```python
from build123d import *

# Parameters (mm, degrees)
F0_R     = 34.798
F1_DEPTH = 6.35
F2_DEPTH = 25.4
F3_DEPTH = 101.6
F4_DEPTH = 101.6


with BuildPart() as f1:
    # F0 (on Front) → F1 (new body)
    with BuildSketch(Plane.XZ):
        Circle(F0_R)
    extrude(amount=F1_DEPTH)

    # F2 (add): a face of the model
    f2_faces = [f1.faces().sort_by_distance(p)[0] for p in [
        (0, -6.35, 0),
    ]]
    extrude(f2_faces, amount=F2_DEPTH)

    # F3 (add): a face of the model
    f3_faces = [f1.faces().sort_by_distance(p)[0] for p in [
        (0, -31.75, 0),
    ]]
    extrude(f3_faces, amount=F3_DEPTH)

    # F4 (add): a face of the model
    f4_faces = [f1.faces().sort_by_distance(p)[0] for p in [
        (0, 0, 0),
    ]]
    extrude(f4_faces, amount=F4_DEPTH)


solid = f1.part
```
Source: CAD feature listing. Evaluate the final solid. Frame: model axes, mm. Round coordinates to 2 decimals unless told otherwise and drop trailing zeros. Loops run counter-clockwise (first coordinate to the right, second up) from the corner with the lowest first, then second, coordinate; pieces in that order, holes last. Notation, with made-up numbers: M 6.5,14.25 L 17.5,14.25 A20 cw 17.5,48.25 Z; hole C 2,87 d9. An arc over 180 degrees is marked long. Use a Markdown table: item, result. Add a question column.
1. Ray query, line 1 along X through (y, z) = (75, 1); line 2 along Z through (x, y) = (-0.5, -121); line 3 along X through (y, z) = (-113, 12). Return the intervals inside material, ascending. Write a range as [from, to].
2. Cut plane C-C, the plane x = 27. Output: boundary loops of the cut face in (y, z), and give its area (3 significant figures).
3. Cut plane B-B, the plane z = 14. Output: boundary loops of the cut face in (x, y), and give its area (3 significant figures).
4. Cut plane A-A, the plane y = -66.5. Output: boundary loops of the cut face in (x, z), and give its area (3 significant figures).
5. Contact query for flat-ended pins moving along their axis: pin 1 (1.5 mm diameter, centred on x = 25, y = -107, fed in from -Z); pin 2 (8 mm diameter, centred on x = -27, y = -25.5, fed in from -Z); pin 3 (5 mm diameter, centred on y = 74, z = -10, fed in from -X). Output: stop coordinate, or through.
Solution:
| question | item | result |
|---|---|---|
| 1 | line 1 | x = [-34.78, 34.78] |
| 1 | line 2 | z = [-34.79, 34.79] |
| 1 | line 3 | x = [-32.66, 32.66] |
| 2 | outline | M -133.35,-21.95 L 101.6,-21.95 L 101.6,21.95 L -133.35,21.95 Z |
| 2 | area | 10,300 mm2 |
| 3 | outline | M -31.86,-133.35 L 31.86,-133.35 L 31.86,101.6 L -31.86,101.6 Z |
| 3 | area | 15,000 mm2 |
| 4 | outline | C 0,0 d69.6 |
| 4 | area | 3,800 mm2 |
| 5 | pin 1 | stops at z = -24.96 |
| 5 | pin 2 | stops at z = -26.11 |
| 5 | pin 3 | stops at x = -33.98 |
